from build123d import *

# Parameters (mm, degrees)
BOSS_EXTRUDE1_DEPTH = 5
SKETCH2_R           = 28.5
BOSS_EXTRUDE2_DEPTH = 45
FILLET1_R           = 20
SKETCH3_R           = 60
BOSS_EXTRUDE3_DEPTH = 6
SKETCH4_R           = 24
CUT_EXTRUDE1_DEPTH  = 36


with BuildPart() as part:
    # Sketch1 → Boss-Extrude1 (new body)
    with BuildSketch(Plane(origin=(0, 0, 0), x_dir=(1, 0, 0), z_dir=(0, 1, 0))):
        with BuildLine():
            ThreePointArc((-45, 39.686269666), (-51.961524227, 30), (-56.869317712, 19.128008337))
            add(Edge.make_bspline(
                [(-11.869317712, -58.814278003), (-485.245924558, -280.156865167), (-56.869317712, 19.128008337)],
                knots=[0, 0, 0, 1, 1, 1], degree=2))
            ThreePointArc((-11.869317712, -58.814278003), (0, -60), (11.869317712, -58.814278003))
            add(Edge.make_bspline(
                [(56.869317712, 19.128008337), (485.245924558, -280.156865167), (11.869317712, -58.814278003)],
                knots=[0, 0, 0, 1, 1, 1], degree=2))
            ThreePointArc((56.869317712, 19.128008337), (51.961524227, 30), (45, 39.686269666))
            add(Edge.make_bspline(
                [(-45, 39.686269666), (0, 560.313730334), (45, 39.686269666)],
                knots=[0, 0, 0, 1, 1, 1], degree=2))
        make_face()
    extrude(amount=BOSS_EXTRUDE1_DEPTH)

    # Sketch2 → Boss-Extrude2 (add)
    with BuildSketch(Plane(origin=(0, 5, 0), x_dir=(1, 0, 0), z_dir=(0, 1, 0))):
        Circle(SKETCH2_R)
    extrude(amount=BOSS_EXTRUDE2_DEPTH)

    # Fillet1
    fillet1_edges = [part.edges().sort_by_distance(p)[0] for p in [
        (-28.5, 50, 0),
    ]]
    fillet(fillet1_edges, radius=FILLET1_R)

    # Sketch3 → Boss-Extrude3 (add)
    with BuildSketch(Plane.XZ):
        Circle(SKETCH3_R)
    extrude(amount=BOSS_EXTRUDE3_DEPTH)

    # Sketch4 → Cut-Extrude1 (cut)
    with BuildSketch(Plane.XZ.offset(6)):
        Circle(SKETCH4_R)
    extrude(amount=-CUT_EXTRUDE1_DEPTH, mode=Mode.SUBTRACT)


solid = part.part
Verification items for the finished model (mm, model axes). A direction names the side the tool comes from. Give positions to 0.01 mm unless a question says otherwise; leave off trailing zeros.
(1) Gauge pin test, flat ends, axial feed: pin 1 (8 mm diameter, centred on y = 1, z = -250, fed in from -X); pin 2 (14.5 mm diameter, centred on x = 5.5, z = -5.5, fed in from -Y); pin 3 (12 mm diameter, centred on x = -188, y = 2, fed in from -Z). Record the tip position at first contact, or that the pin passes through.
(2) Material ranges on line 1 (Z direction, x = 0, y = 6); line 2 (Y direction, x = 1, z = -165.5); line 3 (Y direction, x = -40, z = -21), recorded low to high.
(3) Access from +Z, -Z, +X, -X, +Y, -Y to the whole of each face (thin tool, end or side, straight path). Record for faces 1 (the face through (0, 50, 0)), 2 (the face through (0, 30, 0)).
(4) Mould release check, pull along X, two halves, no side actions. Record for faces 3 (the face through (-23.977, 11.748, 1.055)), 4 (the face through (26.327, 17.325, 10.916)), 5 (the face through (26, -6, 1)): +X half, -X half, draft (parallel to the pull), parting line (faces both ways), or undercut.
Worked out:
1. pin 1: stops at x = -20.5
1. pin 2: stops at y = 30
1. pin 3: stops at z = 71.85
2. line 1: z = -28.5 to -24, 24 to 28.5
2. line 2: y = 0 to 5
2. line 3: y = -6 to 5
3. face 1: +Z, -Z, +X, -X, +Y
3. face 2: -Y
4. face 3: undercut
4. face 4: parting line
4. face 5: draft
